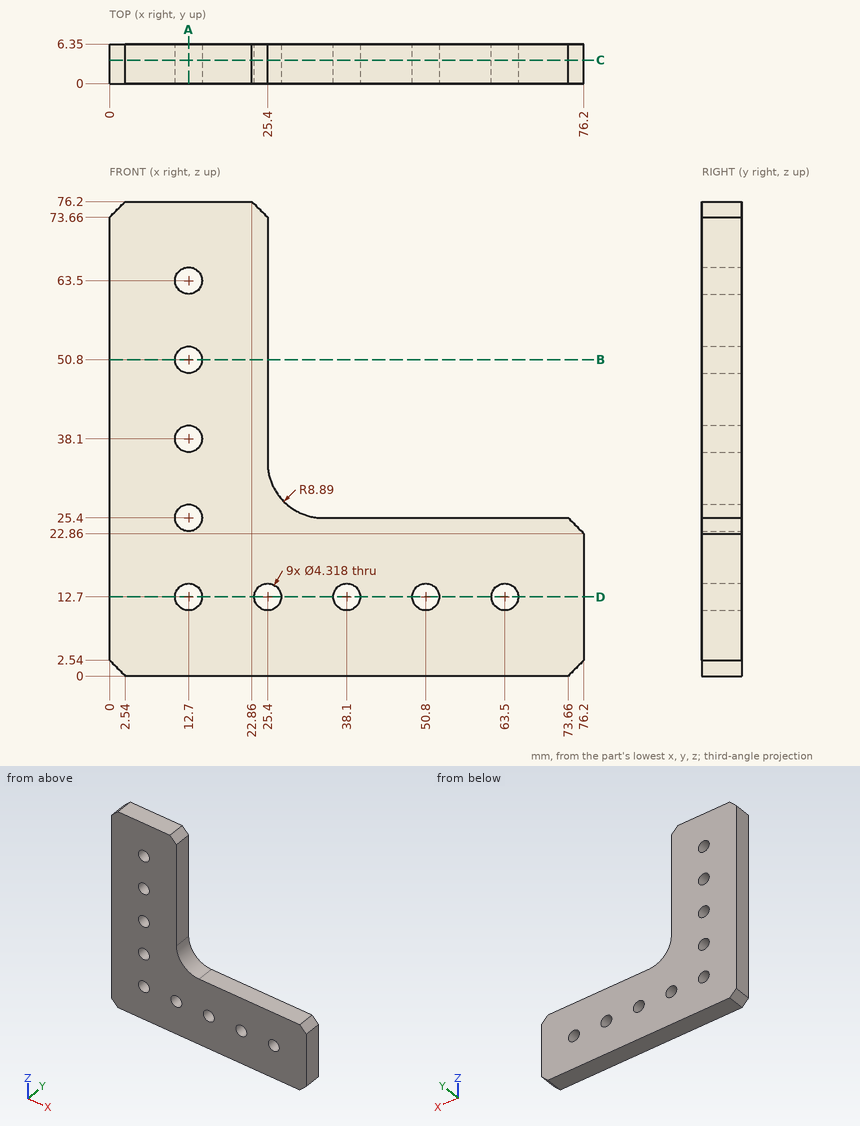
Geometry: see drawing. Coordinates: mm, zero at the bounding-box minimum. Round coordinates to 2 decimals unless told otherwise and drop trailing zeros. Order: outer loops, then holes, each group sorted by start corner. A loop starts at its lowest first (then second) coordinate and runs counter-clockwise, first axis right, second up. Notation, with made-up numbers: (-31.75, 1) -> (23.25, 1) arc R36 cw to (23.25, 35) -> close; hole circle Ø1 at (23, -3.5). An arc over 180 degrees is marked (long way). Answer as CSV lines item,"result".
Item 1: Section D-D, the plane z = 12.7. Return loops of the section in (x, y).
A:
outline,"(0, 0) -> (10.54, 0) -> (10.54, 6.35) -> (0, 6.35) -> close; (14.86, 0) -> (23.24, 0) -> (23.24, 6.35) -> (14.86, 6.35) -> close; (27.56, 0) -> (35.94, 0) -> (35.94, 6.35) -> (27.56, 6.35) -> close; (40.26, 0) -> (48.64, 0) -> (48.64, 6.35) -> (40.26, 6.35) -> close; (52.96, 0) -> (61.34, 0) -> (61.34, 6.35) -> (52.96, 6.35) -> close; (65.66, 0) -> (76.2, 0) -> (76.2, 6.35) -> (65.66, 6.35) -> close"
Item 2: Section C-C, the plane y = 3.75. Count the separate pieces of the cut face and the enclosed holes in it, plus the area to 3 significant figures.
A:
separate pieces,"1"
enclosed holes,"9"
area,"3,090 mm²"
Item 3: Section B-B, the plane z = 50.8. Return loops of the section in (x, y).
A:
outline,"(0, 0) -> (10.54, 0) -> (10.54, 6.35) -> (0, 6.35) -> close; (14.86, 0) -> (25.4, 0) -> (25.4, 6.35) -> (14.86, 6.35) -> close"
Item 4: Section A-A, the plane x = 12.7. Return loops of the section in (y, z).
A:
outline,"(0, 0) -> (6.35, 0) -> (6.35, 10.54) -> (0, 10.54) -> close; (0, 14.86) -> (6.35, 14.86) -> (6.35, 23.24) -> (0, 23.24) -> close; (0, 27.56) -> (6.35, 27.56) -> (6.35, 35.94) -> (0, 35.94) -> close; (0, 40.26) -> (6.35, 40.26) -> (6.35, 48.64) -> (0, 48.64) -> close; (0, 52.96) -> (6.35, 52.96) -> (6.35, 61.34) -> (0, 61.34) -> close; (0, 65.66) -> (6.35, 65.66) -> (6.35, 76.2) -> (0, 76.2) -> close"
Item 5: Pin query (flat end, axial travel): pin 1 Ø5 at (x, z) = (12.7, 12.7) entering from +Y; pin 2 Ø1 at (x, y) = (48, 4) entering from +Z; pin 3 Ø1 at (y, z) = (4.5, 40) entering from +X. Return the tip coordinate at first contact, or that it passes through.
A:
pin 1,"y = 6.35"
pin 2,"z = 25.4"
pin 3,"x = 25.4"
Item 6: Line query: L1, parallel to Z at x = 50.8, y = 3.75; L2, parallel to X at y = 2.25, z = 66.5. Output: solid intervals per line, ascending.
A:
L1,"0 to 10.54, 14.86 to 25.4"
L2,"0 to 25.4"
